Geometry: final body of the model. Coordinates: model frame, mm. A direction names the side the tool comes from. Give positions to 0.01 mm unless a question says otherwise; leave off trailing zeros. Write each loop counter-clockwise with the first axis right and the second up, starting at its lowest first coordinate (ties: lowest second). Pieces come first, ordered by that corner, then holes. Notation, with made-up numbers: M 38.25,87 L 56.25,87 A38 ccw 56.25,126 Z; hole C 65,10.25 d10. An arc over 180 degrees is marked long. One line per question, with ' | ' between items.
from build123d import *

# Parameters (mm, degrees)
F0_W     = 76.2
F0_H     = 76.2
F1_DEPTH = 76.2
F2_W     = 25.4
F2_H     = 25.4
F3_DEPTH = 12.7
F4_R     = 12.7
F5_DEPTH = 12.7
F7_D     = 25.4
F9_DEPTH = 12.7


with BuildPart() as f1:
    # F0 (on Front) → F1 (new body)
    with BuildSketch(Plane.XZ):
        with Locations((-38.1, 49.621367)):
            Rectangle(F0_W, F0_H)
    extrude(amount=F1_DEPTH)

    # F2 (on face) → F3 (join)
    with BuildSketch(Plane.XZ.offset(76.2)):
        with Locations((-38.1, 49.621367)):
            Rectangle(F2_W, F2_H)
    extrude(amount=F3_DEPTH)

    # F4 (on face) → F5 (join)
    with BuildSketch(Plane.YZ):
        with Locations((-38.1, 49.621367)):
            Circle(F4_R)
    extrude(amount=F5_DEPTH)

    # F7 (through all)
    with Locations(Plane.XY.offset(87.721367)):
        with Locations((-38.1, -38.1)):
            Hole(F7_D / 2)

    # F8 (on face) → F9 (join)
    with BuildSketch(Plane(origin=(0, 0, 0), x_dir=(-1, 0, 0), z_dir=(0, 1, 0))):
        Polygon((11.431118, 34.224081), (64.768882, 34.224081), (38.1, 80.415939), align=None)
    extrude(amount=F9_DEPTH)


solid = f1.part
(1) Set-up query: faces 4 (the face through (-51.62, 6.26, 57)), 5 (the face through (-24.95, 6.26, 57.64)), 6 (the face through (-25.4, -82, 49)), 7 (the face through (0, -38, 32)). Return all of +Z, -Z, +X, -X, +Y, -Y with unobstructed straight access to the full face (end or side cutting, diameter ignored); none if empty.
Working result:
face 4: +Z, -X, +Y | face 5: +Z, +X, +Y | face 6: +Z, -Z, +X, -Y | face 7: +X
(2) Draft query along X for faces 1 (the face through (-50.8, -82, 49)), 2 (the face through (-49.832, -42.964, 49.088)), 3 (the face through (-38, -82, 36.921)). Return one class per face: released by +X, released by -X, zero draft, split by the parting line, or undercut.
Working result:
face 1: released by -X | face 2: undercut | face 3: zero draft
(3) Material intervals for L1, parallel to Y at x = -38, z = 49; L2, parallel to Y at x = -38.1, z = 34; L3, parallel to X at y = -41, z = 80.5, sorted ascending. Write a range as [from, to].
Working result:
L1: y = [-88.9, -50.8], [-25.4, 12.7] | L2: y = [-76.2, -50.8], [-25.4, 0] | L3: x = [-76.2, -50.46], [-25.74, 0]
(4) Cut plane C-C, the plane x = -35.5. Return loops of the section in (y, z).
Working result:
outline: M -88.9,36.92 L -76.2,36.92 L -76.2,11.52 L -50.53,11.52 L -50.53,87.72 L -76.2,87.72 L -76.2,62.32 L -88.9,62.32 Z; M -25.67,11.52 L 0,11.52 L 0,34.22 L 12.7,34.22 L 12.7,75.91 L 0,75.91 L 0,87.72 L -25.67,87.72 Z
(5) Cut plane D-D, the plane y = -22. Return loops of the section in (x, z), then the cut area to 3 significant figures.
Working result:
outline: M -76.2,11.52 L 0,11.52 L 0,87.72 L -76.2,87.72 Z | area: 5,810 mm^2
(6) Cut plane A-A, the plane y = -38.1. Return loops of the section in (x, z), then the cut area to 3 significant figures.
Working result:
outline: M -76.2,11.52 L -50.8,11.52 L -50.8,87.72 L -76.2,87.72 Z; M -25.4,11.52 L 0,11.52 L 0,36.92 L 12.7,36.92 L 12.7,62.32 L 0,62.32 L 0,87.72 L -25.4,87.72 Z | area: 4,190 mm^2
(7) First-contact query: P1, Ø10, axis at x = -37.5, y = -81, coming from the +Z side; P2, Ø6, axis at x = -24.5, z = 30, coming from the +Y side; P3, Ø4, axis at x = -53, z = 73.5, coming from the -Y side; P4, Ø14, axis at y = -81, z = 44.5, coming from the +X side. Flat tips, straight axial feed; report the tip coordinate or a pass-through.
Working result:
P1: stops at z = 87.72 | P2: stops at y = 0 | P3: stops at y = -76.2 | P4: stops at x = 0
(8) Cut plane B-B, the plane z = 26.5. Return loops of the section in (x, y), then the cut area to 3 significant figures.
Working result:
outline: M -76.2,-76.2 L 0,-76.2 L 0,0 L -76.2,0 Z; hole C -38.1,-38.1 d25.4 | area: 5,300 mm^2
